```python
from build123d import *

# Parameters (mm, degrees)
SKETCH_W          = 31.5
SKETCH_H          = 58
PAD_DEPTH         = 15
FILLET_R          = 7.5
SKETCH001_W       = 53
SKETCH001_H       = 15
POCKET_DEPTH      = 15.751
POCKET_DEPTH_BACK = 15.751
SKETCH002_W       = 28.5
SKETCH002_H       = 53
POCKET001_DEPTH   = 5
SKETCH003_R       = 1.5
POCKET002_DEPTH   = 15.001
SKETCH004_R       = 2
POCKET003_DEPTH   = 58.001


with BuildPart() as part:
    # Sketch → Pad (new body)
    with BuildSketch(Plane.XY):
        Rectangle(SKETCH_W, SKETCH_H)
    extrude(amount=PAD_DEPTH)

    # Fillet
    fillet_edges = [part.edges().sort_by_distance(p)[0] for p in [
        (15.75, 0, 15),
        (-15.75, 0, 15),
    ]]
    fillet(fillet_edges, radius=FILLET_R)

    # Sketch001 → Pocket (cut, two sides)
    with BuildSketch(Plane.YZ) as pocket_sk:
        with Locations((0, 15)):
            Rectangle(SKETCH001_W, SKETCH001_H)
    extrude(amount=-POCKET_DEPTH, mode=Mode.SUBTRACT)
    extrude(pocket_sk.sketch, amount=POCKET_DEPTH_BACK, mode=Mode.SUBTRACT)

    # Sketch002 (on DatumPlane) → Pocket001 (cut)
    with BuildSketch(Plane.XY.offset(7.5)):
        Rectangle(SKETCH002_W, SKETCH002_H)
    extrude(amount=-POCKET001_DEPTH, mode=Mode.SUBTRACT)

    # Sketch003 → Pocket002 (cut, through all)
    with BuildSketch(Plane.XY):
        with Locations((0, 7.1)):
            Circle(SKETCH003_R)
        Circle(SKETCH003_R)
        with Locations((0, -7.1)):
            Circle(SKETCH003_R)
    extrude(amount=POCKET002_DEPTH, mode=Mode.SUBTRACT)

    # Sketch004 (on Face1 of Pocket002) → Pocket003 (cut, through all)
    with BuildSketch(Plane(origin=(0, 29, 0), x_dir=(-1, 0, 0), z_dir=(0, 1, 0))):
        with Locations((-7, 8.2)):
            Circle(SKETCH004_R)
        with Locations((7, 8.2)):
            Circle(SKETCH004_R)
    extrude(amount=-POCKET003_DEPTH, mode=Mode.SUBTRACT)


solid = part.part
```
Model file for the job. Use its own axes, mm. A direction names the side the tool comes from. Coordinates: 2 decimals unless noted, no trailing zeros. Write each loop counter-clockwise with the first axis right and the second up, starting at its lowest first coordinate (ties: lowest second). Pieces come first, ordered by that corner, then holes. Notation, with made-up numbers: (52, 79.25) - (61, 79.25) arc R30 ccw to (61, 110.25) - close; hole circle Ø6 at (55, 79). An arc over 180 degrees is marked (long way). One line per item, written item: value. Start each with the question number.
1. Slice it at B-B (x = -7). Write the cut outline in (y, z).
2. Slice it at C-C (x = 0). Write the cut outline in (y, z).
3. Tool access for faces 4 (the flat face through (14.25, 0, 5)), 5 (the flat face through (15, 0, 7.5)), 6 (the cylindrical face through (-13.611, 27.768, 12.745)): list every direction of +Z, -Z, +X, -X, +Y, -Y with a clear straight run to the whole face (end or side of a thin tool).
4. Flat gauge pins, fed straight in: pin 1 (8 mm diameter, centred on x = 2.5, y = 0.5, fed in from +Z); pin 2 (1.2 mm diameter, centred on x = -15.5, y = -8, fed in from +Z). Where does each tip first touch, or does it go through?
5. Slice it at D-D (z = 3.5). Write the cut outline in (x, y).
6. Slice it at A-A (y = -7.1). Write the cut outline in (x, z), plus the area to 4 significant figures.
7. Mould opens along Y. For faces 1 (the flat face through (15.75, 0, 4)), 2 (the flat face through (-14.25, 0, 5)), 3 (the flat face through (0, 29, 7)) say: released by +Y, released by -Y, zero draft, split by the parting line, or undercut.
8. Probe line 1 (Y direction, x = 0, z = 1.5); line 2 (Y direction, x = 1, z = 9.5); line 3 (X direction, y = 0, z = 1.7). List the from-to ranges inside material, lowest first. Write a range as from..to.
Answers below:
1. outline: (-29, 0) - (29, 0) - (29, 6.2) - (26.5, 6.2) - (26.5, 2.5) - (-26.5, 2.5) - (-26.5, 6.2) - (-29, 6.2) - close; (-29, 10.2) - (-26.5, 10.2) - (-26.5, 15) - (-29, 15) - close; (26.5, 10.2) - (29, 10.2) - (29, 15) - (26.5, 15) - close
2. outline: (-29, 0) - (-8.6, 0) - (-8.6, 2.5) - (-26.5, 2.5) - (-26.5, 15) - (-29, 15) - close; (-5.6, 0) - (-1.5, 0) - (-1.5, 2.5) - (-5.6, 2.5) - close; (1.5, 0) - (5.6, 0) - (5.6, 2.5) - (1.5, 2.5) - close; (8.6, 0) - (29, 0) - (29, 15) - (26.5, 15) - (26.5, 2.5) - (8.6, 2.5) - close
3. face 4: +Z
3. face 5: +Z, +X, -X
3. face 6: +Z, -X, +Y, -Y
4. pin 1: stops at z = 2.5
4. pin 2: stops at z = 7.5
5. outline: (-15.75, -29) - (15.75, -29) - (15.75, 29) - (-15.75, 29) - close; hole (-14.25, -26.5) - (14.25, -26.5) - (14.25, 26.5) - (-14.25, 26.5) - close
6. outline: (-15.75, 0) - (-1.5, 0) - (-1.5, 2.5) - (-14.25, 2.5) - (-14.25, 7.5) - (-15.75, 7.5) - close; (1.5, 0) - (15.75, 0) - (15.75, 7.5) - (14.25, 7.5) - (14.25, 2.5) - (1.5, 2.5) - close
6. area: 86.25 mm^2
7. face 1: zero draft
7. face 2: undercut
7. face 3: released by +Y
8. line 1: y = -29..-8.6, -5.6..-1.5, 1.5..5.6, 8.6..29
8. line 2: y = -29..-26.5, 26.5..29
8. line 3: x = -15.75..-1.5, 1.5..15.75
